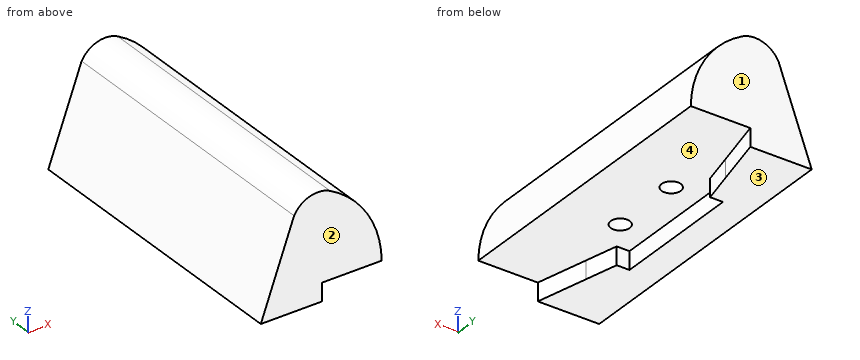
from build123d import *

# Parameters (mm, degrees)
BOSS_EXTRUDE1_DEPTH = 50
CUT_EXTRUDE1_DEPTH  = 50
SKETCH3_R           = 1.6
CUT_EXTRUDE2_DEPTH  = 15
SKETCH6_R           = 1.6
CUT_EXTRUDE4_DEPTH  = 3
SKETCH7_W           = 1.666520658
SKETCH7_H           = 50
CUT_EXTRUDE5_DEPTH  = 3
CUT_EXTRUDE6_DEPTH  = 3


with BuildPart() as part:
    # Sketch1 → Boss-Extrude1 (new body)
    with BuildSketch(Plane(origin=(0, 0, 0), x_dir=(1, 0, 0), z_dir=(0, 1, 0))):
        with BuildLine():
            Line((13.159597133, 18.793852416), (-6.840402867, 18.793852416))
            Line((-6.840402867, 18.793852416), (0, 0))
            ThreePointArc((0, 0), (10.472132847, 6.671484404), (13.159597133, 18.793852416))
        make_face()
    extrude(amount=BOSS_EXTRUDE1_DEPTH)

    # Sketch5 → Cut-Extrude1 (cut)
    with BuildSketch(Plane(origin=(0, 50, 0), x_dir=(1, 0, 0), z_dir=(0, 1, 0))):
        with BuildLine():
            ThreePointArc((4.765485224, 1.634621553), (1.372703273, 1.322660653), (-1.265925556, 3.478101879))
            Line((-1.265925556, 3.478101879), (0, 0))
            ThreePointArc((0, 0), (2.446582795, 0.63119464), (4.765485224, 1.634621553))
        make_face()
    extrude(amount=-CUT_EXTRUDE1_DEPTH, mode=Mode.SUBTRACT)

    # Sketch3 → Cut-Extrude2 (cut)
    with BuildSketch(Plane(origin=(0, 0, -18.793852416), x_dir=(-1, 0, 0), z_dir=(0, 0, -1))):
        with Locations((-3.159597133, 19)):
            Circle(SKETCH3_R)
        with Locations((-3.159597133, 31)):
            Circle(SKETCH3_R)
    extrude(amount=-CUT_EXTRUDE2_DEPTH, mode=Mode.SUBTRACT)

    # Sketch6 → Cut-Extrude4 (cut)
    with BuildSketch(Plane(origin=(0, 0, -18.793852416), x_dir=(-1, 0, 0), z_dir=(0, 0, -1))):
        Polygon((0.945619298, 31), (0.737883126, 31.899804217), (-0.208721658, 36), (-1.45536469, 41.399804217), (-3.440876334, 50), (-7.546092765, 50), (-13.159597133, 50), (-13.159597133, 0), (-7.546092765, 0), (-3.440876334, 0), (-1.45536469, 8.600195783), (-0.208721658, 14), (0.737883126, 18.100195783), (0.945619298, 19), align=None)
        with Locations((-3.159597133, 19)):
            Circle(SKETCH6_R, mode=Mode.SUBTRACT)
        with Locations((-3.159597133, 31)):
            Circle(SKETCH6_R, mode=Mode.SUBTRACT)
        Polygon((-0.208721658, 36), (0.737883126, 31.899804217), (0.945619298, 31), (0.945619298, 36), align=None)
        Polygon((0.945619298, 14), (0.945619298, 19), (0.737883126, 18.100195783), (-0.208721658, 14), align=None)
    extrude(amount=-CUT_EXTRUDE4_DEPTH, mode=Mode.SUBTRACT)

    # Sketch7 → Cut-Extrude5 (cut)
    with BuildSketch(Plane(origin=(0, 0, -18.793852416), x_dir=(-1, 0, 0), z_dir=(0, 0, -1))):
        with Locations((-13.992857462, 25)):
            Rectangle(SKETCH7_W, SKETCH7_H)
    extrude(amount=-CUT_EXTRUDE5_DEPTH, mode=Mode.SUBTRACT)

    # Sketch6_5 → Cut-Extrude6 (cut)
    with BuildSketch(Plane(origin=(0, 0, -18.793852416), x_dir=(-1, 0, 0), z_dir=(0, 0, -1))):
        Polygon((1.945619298, 36), (1.945619298, 14), (0.945619298, 14), (0.945619298, 19), (0.945619298, 31), (0.945619298, 36), align=None)
    extrude(amount=-CUT_EXTRUDE6_DEPTH, mode=Mode.SUBTRACT)


solid = part.part
Read the model definition and answer for the solid it produces. Units are mm, in the model's axes. Face numbers are marked on the shaded views. Round coordinates to 2 decimals unless told otherwise and drop trailing zeros. Write each loop counter-clockwise with the first axis right and the second up, starting at its lowest first coordinate (ties: lowest second). Pieces come first, ordered by that corner, then holes.
1. Straight lines are drawn through the part: L1, parallel to Y at x = 2, z = -5.5; L2, parallel to Y at x = 2.5, z = -4.75; L3, parallel to Z at x = 12, y = 48.5. For each, find the intervals that lie inside material, in ascending order.
2. The part is cut by section C-C, the plane z = -6.25. Determine the outline of the cut face in (x, y), then the cut area to 3 significant figures.
3. The part is cut by section B-B, the plane z = -14. Determine the outline of the cut face in (x, y), then the cut area to 3 significant figures.
4. The part is cut by section D-D, the plane y = 18.5. Determine the outline of the cut face in (x, z), then the cut area to 3 significant figures.
5. The part is cut by section A-A, the plane y = 31. Determine the outline of the cut face in (x, z), then the cut area to 3 significant figures.
6. Determine the mould class of the marked faces 1, 2, 3 and 4 for opening direction Y: pulls with the +Y half, pulls with the -Y half, needs draft (parallel to the pull), parting line crosses it, or undercut.
7. Given pin 1 Ø3 at (y, z) = (28.5, -13.5) entering from -X; pin 2 Ø3 at (y, z) = (38.5, -16) entering from -X; pin 3 Ø1.1 at (x, z) = (-0.5, -17.5) entering from -Y; pin 4 Ø2.5 at (x, y) = (3.5, 19.5) entering from -Z, each flat-ended and moving along its own axis, determine where each tip first touches the part or whether it passes through.
Values:
1. L1: y = 0 to 17.9, 20.1 to 29.9, 32.1 to 50
1. L2: y = 0 to 17.54, 20.46 to 29.54, 32.46 to 50
1. L3: z = -15.79 to -9.37
2. outline: (-2.27, 0) - (10.17, 0) - (10.17, 50) - (-2.27, 50) - close; hole circle Ø3.2 at (3.16, 19); hole circle Ø3.2 at (3.16, 31)
2. area: 606 mm2
3. outline: (-5.1, 0) - (13.29, 0) - (13.29, 50) - (-5.1, 50) - close; hole circle Ø3.2 at (3.16, 19); hole circle Ø3.2 at (3.16, 31)
3. area: 903 mm2
4. outline: (-6.84, -18.79) - (-1.95, -18.79) - (-1.95, -15.79) - (1.64, -15.79) - (1.64, -3.79) - (4.68, -3.79) - (4.68, -15.79) - (13.41, -15.79) arc R16.22 ccw to (4.77, -1.63) arc R4.5 ccw to (-1.27, -3.48) - close
4. area: 176 mm2
5. outline: (-6.84, -18.79) - (-1.95, -18.79) - (-1.95, -15.79) - (1.56, -15.79) - (1.56, -3.79) - (4.76, -3.79) - (4.76, -15.79) - (13.41, -15.79) arc R16.22 ccw to (4.77, -1.63) arc R4.5 ccw to (-1.27, -3.48) - close
5. area: 174 mm2
6. face 1: pulls with the +Y half
6. face 2: pulls with the -Y half
6. face 3: needs draft
6. face 4: undercut
7. pin 1: stops at x = -5.46
7. pin 2: stops at x = -6.37
7. pin 3: stops at y = 0
7. pin 4: stops at z = -15.79
